Design review of the part built by this model. Coordinates are the model's own, in mm. Coordinates: 2 decimals unless noted, no trailing zeros. Write each loop counter-clockwise with the first axis right and the second up, starting at its lowest first coordinate (ties: lowest second). Pieces come first, ordered by that corner, then holes.
Q1. Take a section at B-B (x = 88.9). Give the boundary of the cut face in (y, z).
Q2. For probe 1 along Z at (x, y) = (88.9, -4.5); probe 2 along Y at (x, z) = (25, 7); probe 3 along X at (y, z) = (-2.25, 21.5), list the stretches that pass through material, from the lowest coordinate up.
Q3. Insertion check: pin 1 (7.5 mm diameter, centred on x = 330.2, z = 25.4, fed in from +Y); pin 2 (2 mm diameter, centred on y = -4.5, z = 20.5, fed in from +X); pin 3 (1.5 mm diameter, centred on y = -3.5, z = 7, fed in from +X); pin 4 (3 mm diameter, centred on x = 25.4, y = -3.175, fed in from +Z). Each pin has a flat end and moves straight along its axis. Give the tip position at first contact, or say it passes through.
Q4. Take a section at A-A (x = 256.54). Give the boundary of the cut face in (y, z), and give its area (3 significant figures).
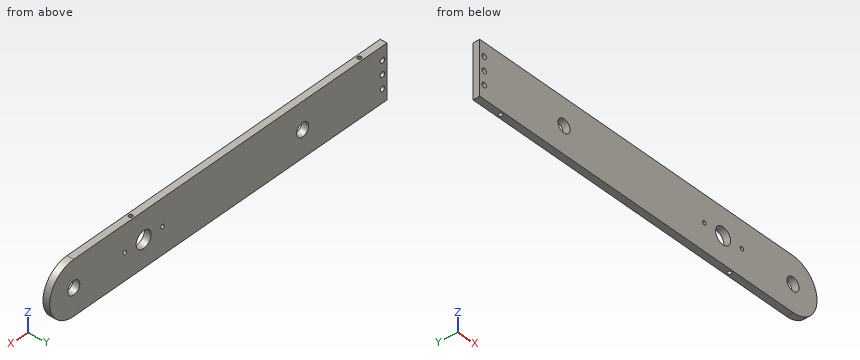
```python
from build123d import *

# Parameters (mm, degrees)
F0_R      = 6.35
F0_R_2    = 1.7907
F0_R_3    = 7.9375
F1_DEPTH  = 6.35
F2_D      = 4.7625
F2_DEPTH  = 12.7
F2_TIP    = 1.4307993491
F3_D      = 4.7625
F3_DEPTH  = 12.7
F3_TIP    = 1.4307993491
F4_D      = 4.7625
F4_DEPTH  = 12.7
F4_TIP    = 1.4307993491
F6_D      = 3.571875
F6_DEPTH  = 12.7
F6_TIP    = 1.0730995118
F7_D      = 3.571875
F7_DEPTH  = 12.7
F7_TIP    = 1.0730995118
F9_D      = 3.571875
F9_DEPTH  = 6.35
F9_TIP    = 1.0730995118
F10_D     = 3.571875
F10_DEPTH = 6.35
F10_TIP   = 1.0730995118


with BuildPart() as f1:
    # F0 (on Front) → F1 (new body)
    with BuildSketch(Plane.XZ):
        with BuildLine():
            Line((0, 50.8), (0, 0))
            Line((0, 0), (330.2, 0))
            ThreePointArc((330.2, 0), (355.6, 25.4), (330.2, 50.8))
            Line((330.2, 50.8), (0, 50.8))
        make_face()
        with Locations((88.9, 25.4)):
            Circle(F0_R, mode=Mode.SUBTRACT)
        with Locations((236.7026, 25.4)):
            Circle(F0_R_2, mode=Mode.SUBTRACT)
        with Locations((256.54, 25.4)):
            Circle(F0_R_3, mode=Mode.SUBTRACT)
        with BuildLine():
            ThreePointArc((278.1681, 25.4), (276.3774, 23.6093), (274.5867, 25.4))
            ThreePointArc((274.5867, 25.4), (276.3774, 27.1907), (278.1681, 25.4))
        make_face(mode=Mode.SUBTRACT)
        with Locations((330.2, 25.4)):
            Circle(F0_R, mode=Mode.SUBTRACT)
    extrude(amount=F1_DEPTH)

    # F2
    with Locations(Plane(origin=(0, 0, 0), x_dir=(1, 0, 0), z_dir=(0, 1, 0))):
        with Locations((4.7625, -25.4)):
            Hole(F2_D / 2, depth=F2_DEPTH)
            with Locations((0, 0, -(F2_DEPTH + F2_TIP / 2))):  # 118° drill point
                Cone(0, F2_D / 2, F2_TIP, mode=Mode.SUBTRACT)

    # F3
    with Locations(Plane(origin=(0, 0, 0), x_dir=(1, 0, 0), z_dir=(0, 1, 0))):
        with Locations((4.7625, -12.7)):
            Hole(F3_D / 2, depth=F3_DEPTH)
            with Locations((0, 0, -(F3_DEPTH + F3_TIP / 2))):  # 118° drill point
                Cone(0, F3_D / 2, F3_TIP, mode=Mode.SUBTRACT)

    # F4
    with Locations(Plane(origin=(0, 0, 0), x_dir=(1, 0, 0), z_dir=(0, 1, 0))):
        with Locations((4.7625, -38.1)):
            Hole(F4_D / 2, depth=F4_DEPTH)
            with Locations((0, 0, -(F4_DEPTH + F4_TIP / 2))):  # 118° drill point
                Cone(0, F4_D / 2, F4_TIP, mode=Mode.SUBTRACT)

    # F6
    with Locations(Plane(origin=(0, 0, 0), x_dir=(1, 0, 0), z_dir=(0, 0, -1))):
        with Locations((266.7, 3.175)):
            Hole(F6_D / 2, depth=F6_DEPTH)
            with Locations((0, 0, -(F6_DEPTH + F6_TIP / 2))):  # 118° drill point
                Cone(0, F6_D / 2, F6_TIP, mode=Mode.SUBTRACT)

    # F7
    with Locations(Plane(origin=(0, 0, 0), x_dir=(1, 0, 0), z_dir=(0, 0, -1))):
        with Locations((25.4, 3.175)):
            Hole(F7_D / 2, depth=F7_DEPTH)
            with Locations((0, 0, -(F7_DEPTH + F7_TIP / 2))):  # 118° drill point
                Cone(0, F7_D / 2, F7_TIP, mode=Mode.SUBTRACT)

    # F9
    with Locations(Plane.XY.offset(50.8)):
        with Locations((266.7, -3.175)):
            Hole(F9_D / 2, depth=F9_DEPTH)
            with Locations((0, 0, -(F9_DEPTH + F9_TIP / 2))):  # 118° drill point
                Cone(0, F9_D / 2, F9_TIP, mode=Mode.SUBTRACT)

    # F10
    with Locations(Plane.XY.offset(50.8)):
        with Locations((25.4, -3.175)):
            Hole(F10_D / 2, depth=F10_DEPTH)
            with Locations((0, 0, -(F10_DEPTH + F10_TIP / 2))):  # 118° drill point
                Cone(0, F10_D / 2, F10_TIP, mode=Mode.SUBTRACT)


solid = f1.part
```
Response:
1. outline: (-6.35, 0) - (0, 0) - (0, 19.05) - (-6.35, 19.05) - close; (-6.35, 31.75) - (0, 31.75) - (0, 50.8) - (-6.35, 50.8) - close
2. probe 1: z = 0 to 19.05, 31.75 to 50.8
2. probe 2: y = -6.35 to -4.92, -1.43 to 0
2. probe 3: x = 0 to 83.89, 93.91 to 249.63, 263.45 to 325.19, 335.21 to 355.3
3. pin 1: passes through
3. pin 2: stops at x = 355.3
3. pin 3: stops at x = 348.47
3. pin 4: stops at z = 44.28
4. outline: (-6.35, 0) - (0, 0) - (0, 17.46) - (-6.35, 17.46) - close; (-6.35, 33.34) - (0, 33.34) - (0, 50.8) - (-6.35, 50.8) - close
4. area: 222 mm2
